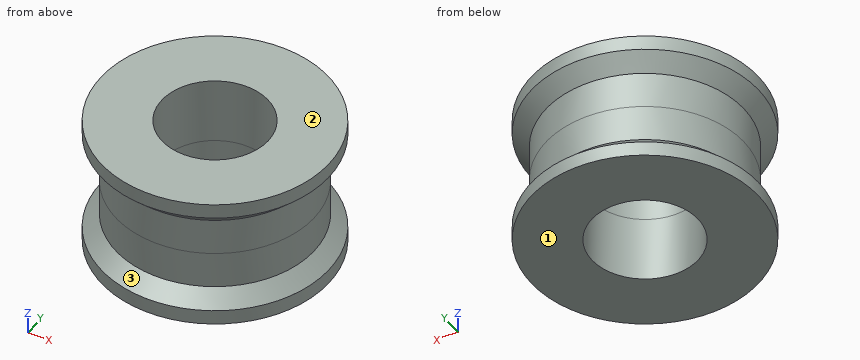
from build123d import *

# Parameters (mm, degrees)
SKETCH1_R           = 7.75
SKETCH1_R_2         = 3.625
BOSS_EXTRUDE1_DEPTH = 1
SKETCH2_R           = 6.75
SKETCH2_R_2         = 3.625
BOSS_EXTRUDE2_DEPTH = 3.5
CHAMFER1_SIZE       = 1


with BuildPart() as part:
    # Sketch1 → Boss-Extrude1 (new body)
    with BuildSketch(Plane.XY):
        Circle(SKETCH1_R)
        Circle(SKETCH1_R_2, mode=Mode.SUBTRACT)
    extrude(amount=BOSS_EXTRUDE1_DEPTH)

    # Sketch2 → Boss-Extrude2 (add)
    with BuildSketch(Plane.XY.offset(1)):
        Circle(SKETCH2_R)
        Circle(SKETCH2_R_2, mode=Mode.SUBTRACT)
    extrude(amount=BOSS_EXTRUDE2_DEPTH)

    # Chamfer1
    chamfer1_edges = [part.edges().sort_by_distance(p)[0] for p in [
        (-6.75, 0, 1),
    ]]
    chamfer(chamfer1_edges, length=CHAMFER1_SIZE - 0.0001)  # a hair under: the kernel refuses the full size

    # Mirror5: part across plane


with BuildPart() as part_1:
    add(part.part)
    add(part.part.mirror(Plane.XY.offset(4.5)))


solid = part_1.part
Build history of the part. All positions in model axes, mm. Face numbers are marked on the shaded views. Coordinates: 2 decimals unless noted, no trailing zeros. Order: outer loops, then holes, each group sorted by start corner. A loop starts at its lowest first (then second) coordinate and runs counter-clockwise, first axis right, second up. Notation, with made-up numbers: (12.25, 36) - (21.25, 36) arc R28 ccw to (21.25, 61) - close; hole circle Ø10 at (2, 58). An arc over 180 degrees is marked (long way). Write item = value, one per line. Start each with the question number.
1) Saw through at D-D on z = 1.25. Write the cut outline in (x, y) (3 decimals), then the cut area to 3 significant figures.
2) Wall check: line 1 along Y through (x, z) = (0, 3.05) (3 decimals); line 2 along Y through (x, z) = (0, 0.9) (3 decimals); line 3 along X through (y, z) = (-2, 1.75). Give the ranges that are in metal, low to high. Write a range as from..to.
3) Two-plate mould, pull along Z, no slides. Class the marked faces 1, 2 and 3: pulls with the +Z half, pulls with the -Z half, needs draft (parallel to the pull), parting line crosses it, or undercut.
4) Flat gauge pins, fed straight in: pin 1 Ø1 at (x, z) = (3.5, 3) entering from -Y; pin 2 Ø6 at (x, y) = (0, 0) entering from +Z; pin 3 Ø5 at (x, z) = (-3, 2) entering from +Y; pin 4 Ø5 at (y, z) = (5, 6.5) entering from +X. Where does each tip first touch, or does it go through?
5) Saw through at C-C on z = 2.25. Write the cut outline in (x, y) (3 decimals).
From the geometry:
q1.outline = circle Ø15 at (0, 0); hole circle Ø7.25 at (0, 0)
q1.area = 135 mm^2
q2.line_1 = -6.75..-3.625, 3.625..6.75
q2.line_2 = -7.75..-3.625, 3.625..7.75
q2.line_3 = -6.71..-3.02, 3.02..6.71
q3.face_1 = pulls with the -Z half
q3.face_2 = pulls with the +Z half
q3.face_3 = undercut
q4.pin_1 = -6.05
q4.pin_2 = through
q4.pin_3 = 7.72
q4.pin_4 = 7.15
q5.outline = circle Ø13.5 at (0, 0); hole circle Ø7.25 at (0, 0)
